Check sheet for the modelled part. Datum: model origin and axes. Units: mm. A direction names the side the tool comes from. Round coordinates to 2 decimals unless told otherwise and drop trailing zeros. Order: outer loops, then holes, each group sorted by start corner. A loop starts at its lowest first (then second) coordinate and runs counter-clockwise, first axis right, second up.
Q1. Mould release check, pull along Z, two halves, no side actions. Record for faces 4 (the cylindrical face through (35.07, 7.81, -1.73)), 5 (the flat face through (0, 0.1, 3.4)), 6 (the cylindrical face through (19.72, 2.64, 59.94)): +Z half, -Z half, draft (parallel to the pull), parting line (faces both ways), or undercut.
Q2. Set-up check for faces 1 (the flat face through (15, 10, -10)), 2 (the flat face through (40, -0.1, 3.4)), 3 (the flat face through (25, -10, -10)): record each of +Z, -Z, +X, -X, +Y, -Y from which the full face is reachable in a straight line by a thin tool's end or side.
Q3. Depth check by flat-ended pin: P1, Ø6, axis at y = -26, z = 30, coming from the -X side; P2, Ø6, axis at x = 32, y = -21, coming from the -Z side; P3, Ø4, axis at x = 12.5, y = 9.5, coming from the -Z side. Enter the tip coordinate at first touch or a pass-through.
Q4. Cross-section at D-D on x = 21. Record the cut outline in (y, z).
Q5. Cross-section at C-C on x = 28. Record the cut outline in (y, z), then the cut area to 3 significant figures.
Q6. Cross-section at A-A on z = 0. Record the cut outline in (x, y), then the cut area to 3 significant figures.
Q7. Scan lines: probe 1 along Y at (x, z) = (30, 0); probe 2 along Z at (x, y) = (31.5, -2.5); probe 3 along X at (y, z) = (7, 44). Record each from-to range of solid material in increasing order.
from build123d import *

# Parameters (mm, degrees)
SKETCH2_R           = 60
BOSS_EXTRUDE1_DEPTH = 40
SKETCH3_R           = 50
CUT_EXTRUDE1_DEPTH  = 15
CUT_EXTRUDE2_START  = -15
SKETCH4_R           = 50
CUT_EXTRUDE2_DEPTH  = 15
SKETCH5_R           = 8
BOSS_EXTRUDE2_DEPTH = 15
BOSS_EXTRUDE3_START = 15
SKETCH6_R           = 8
BOSS_EXTRUDE3_DEPTH = 15
SKETCH7_R           = 3
CUT_EXTRUDE3_DEPTH  = 40
FILLET2_R           = 5


with BuildPart() as part:
    # Sketch2 → Boss-Extrude1 (new body)
    with BuildSketch(Plane(origin=(0, 0, 0), x_dir=(0, 0, -1), z_dir=(1, 0, 0))):
        Circle(SKETCH2_R)
    extrude(amount=BOSS_EXTRUDE1_DEPTH)

    # Sketch3 → Cut-Extrude1 (cut)
    with BuildSketch(Plane(origin=(40, 0, 0), x_dir=(0, 0, -1), z_dir=(1, 0, 0))):
        Circle(SKETCH3_R)
    extrude(amount=-CUT_EXTRUDE1_DEPTH, mode=Mode.SUBTRACT)

    # Sketch4 → Cut-Extrude2 (cut)
    with BuildSketch(Plane.ZY.offset(CUT_EXTRUDE2_START)):
        with Locations(Location((0, 0, 0), (0, 0, 180))):
            Circle(SKETCH4_R)
    extrude(amount=CUT_EXTRUDE2_DEPTH, mode=Mode.SUBTRACT)

    # Sketch5 → Boss-Extrude2 (add)
    with BuildSketch(Plane.ZY.offset(-15)):
        Circle(SKETCH5_R)
    extrude(amount=BOSS_EXTRUDE2_DEPTH)

    # Sketch6 → Boss-Extrude3 (add)
    with BuildSketch(Plane(origin=(25, 0, 0), x_dir=(0, 0, -1), z_dir=(1, 0, 0)).offset(BOSS_EXTRUDE3_START)):
        with Locations(Location((0, 0, 0), (0, 0, 180))):
            Circle(SKETCH6_R)
    extrude(amount=-BOSS_EXTRUDE3_DEPTH)

    # Sketch7 → Cut-Extrude3 (cut)
    with BuildSketch(Plane(origin=(40, 0, 0), x_dir=(0, 0, -1), z_dir=(1, 0, 0))):
        Circle(SKETCH7_R)
    extrude(amount=-CUT_EXTRUDE3_DEPTH, mode=Mode.SUBTRACT)

    # Fillet2
    fillet2_edges = [part.edges().sort_by_distance(p)[0] for p in [
        (15, 0, -8),
        (25, 0, -8),
    ]]
    fillet(fillet2_edges, radius=FILLET2_R)


solid = part.part
Results found:
1. face 4: undercut
1. face 5: draft
1. face 6: parting line
2. face 1: -X
2. face 2: +Z, -Z, +X, +Y, -Y
2. face 3: +X
3. P1: stops at x = 15
3. P2: stops at z = -57.24
3. P3: stops at z = -59.53
4. outline: circle Ø120 at (0, 0); hole circle Ø6 at (0, 0)
5. outline: circle Ø120 at (0, 0); circle Ø16.83 at (0, 0); hole circle Ø100 at (0, 0); hole circle Ø6 at (0, 0)
5. area: 3,650 mm2
6. outline: (0, -60) - (40, -60) - (40, -50) - (25, -50) - (25, -13) arc R5 cw to (30, -8) - (40, -8) - (40, -3) - (0, -3) - (0, -8) - (10, -8) arc R5 cw to (15, -13) - (15, -50) - (0, -50) - close; (0, 3) - (40, 3) - (40, 8) - (30, 8) arc R5 cw to (25, 13) - (25, 50) - (40, 50) - (40, 60) - (0, 60) - (0, 50) - (15, 50) - (15, 13) arc R5 cw to (10, 8) - (0, 8) - close
6. area: 2,060 mm2
7. probe 1: y = -60 to -50, -8 to -3, 3 to 8, 50 to 60
7. probe 2: z = -59.95 to -49.94, -7.6 to -1.66, 1.66 to 7.6, 49.94 to 59.95
7. probe 3: x = 15 to 25
